from build123d import *

# Parameters (mm, degrees)
F1_DEPTH = 3.8
F2_DEPTH = 7.6
F3_R     = 7
F4_R     = 3
F5_R     = 4
F6_R     = 1.7


with BuildPart() as f1:
    # F0 (on Front) → F1 (new body)
    with BuildSketch(Plane.XZ):
        with BuildLine():
            Line((19.1431716898, 4.4253403938), (8.1440456616, 19.750261103))
            Line((8.1440456616, 19.750261103), (-6.1453692615, 19.750261103))
            add(Edge.make_bspline(
                [(-6.1453692615, 19.750261103), (-9.4334975883, 18.3276780648), (-20.4694799737, 9.4077816301), (-28.441204782, -7.9211202874), (-28.3713925064, -15.033986271), (-24.9090821352, -17.6588842502), (-22.1613161266, -18.3001520287)],
                knots=[0, 0, 0, 0, 0.3043807241, 0.630499808, 0.8116691041, 1, 1, 1, 1], degree=3))
            add(Edge.make_bspline(
                [(-22.1613161266, -18.3001520287), (-20.4320557503, -18.7037231321), (-13.2463438928, -20.672034694), (-7.2728786379, -21.7751605126)],
                knots=[0, 0, 0, 0, 14.676670933, 14.676670933, 14.676670933, 14.676670933], degree=3))
            add(Edge.make_bspline(
                [(-7.2728786379, -21.7751605126), (-10.7580149359, -20.0565494265), (-8.7832123206, -14.063103822), (-8.03378309, -11.3945532964), (-9.0233562514, -8.6834942922)],
                knots=[0, 0, 0, 0, 0.5245717937, 1, 1, 1, 1], degree=3))
            add(Edge.make_bspline(
                [(-9.0233562514, -8.6834942922), (-10.6191516402, -5.3268720907), (-10.1119981872, -0.4332128436), (-8.8609410373, 1.4029428946), (-3.6260034076, 1.6703835883), (-3.5176839858, 0), (-3.8980361515, -1.1065827018)],
                knots=[0, 0, 0, 0, 0.3686579414, 0.5465668413, 0.8102724675, 1, 1, 1, 1], degree=3))
            ThreePointArc((-3.8980361515, -1.1065827018), (0.6821136218, 1.3926973088), (5.0296685697, -1.4922530361))
            add(Edge.make_bspline(
                [(8.4968951944, -8.8667105614), (10.512974474, -6.6020334922), (10.6178822415, 0.1333355699), (9.2147437469, 1.7017312358), (5.6166367294, 1.6619292411), (4.4507364715, 0.9827180402), (4.4928646091, -0.16227164), (5.0296685697, -1.4922530361)],
                knots=[0, 0, 0, 0, 0.3364900582, 0.4892530829, 0.6935980051, 0.8097848409, 0.9832063696, 0.9832063696, 0.9832063696, 0.9832063696], degree=3))
            add(Edge.make_bspline(
                [(8.4968951944, -8.8667105614), (8.93450925, -9.375769436), (10.8149022533, -11.1384536985), (13.7340780615, -11.7891050671), (15.0382904123, -11.7891050671)],
                knots=[0.3188114686, 0.3188114686, 0.3188114686, 0.3188114686, 0.5009211334, 1, 1, 1, 1], degree=3))
            Line((15.0382904123, -11.7891050671), (19.1431716898, -11.7891050671))
            Line((19.1431716898, -11.7891050671), (19.1431716898, 4.4253403938))
        make_face()
        with BuildLine():
            ThreePointArc((-22.1613161266, -14.6834942922), (-25.1613161266, -11.6834942922), (-22.1613161266, -8.6834942922))
            Line((-22.1613161266, -8.6834942922), (-14.628011294, -8.6834942922))
            ThreePointArc((-14.628011294, -8.6834942922), (-11.628011294, -11.6834942922), (-14.628011294, -14.6834942922))
            Line((-14.628011294, -14.6834942922), (-22.1613161266, -14.6834942922))
        make_face(mode=Mode.SUBTRACT)
        with BuildLine():
            ThreePointArc((3.2729445693, 16.7312547565), (6.2729445693, 13.7312547565), (3.2729445693, 10.7312547565))
            Line((3.2729445693, 10.7312547565), (-4.2603602633, 10.7312547565))
            ThreePointArc((-4.2603602633, 10.7312547565), (-7.2603602633, 13.7312547565), (-4.2603602633, 16.7312547565))
            Line((-4.2603602633, 16.7312547565), (3.2729445693, 16.7312547565))
        make_face(mode=Mode.SUBTRACT)
    extrude(amount=F1_DEPTH)

    # F0 (on Front) → F2 (join)
    with BuildSketch(Plane.XZ):
        with BuildLine():
            add(Edge.make_bspline(
                [(-7.2728786379, -21.7751605126), (-10.7580149359, -20.0565494265), (-8.7832123206, -14.063103822), (-8.03378309, -11.3945532964), (-9.0233562514, -8.6834942922)],
                knots=[0, 0, 0, 0, 0.5245717937, 1, 1, 1, 1], degree=3))
            add(Edge.make_bspline(
                [(-7.2728786379, -21.7751605126), (-3.8634845801, -22.4047767321), (-0.848995576, -22.7525474742), (0.5306684761, -22.3666733306)],
                knots=[14.676670933, 14.676670933, 14.676670933, 14.676670933, 23.053476109, 23.053476109, 23.053476109, 23.053476109], degree=3))
            ThreePointArc((0.5306684761, -22.3666733306), (1.3315647917, -21.7109648486), (1.3916492908, -20.6776312264))
            Line((1.3916492908, -20.6776312264), (-4.2720503639, -5.4112309833))
            ThreePointArc((-4.2720503639, -5.4112309833), (-4.5685146727, -3.2168998843), (-3.8980361515, -1.1065827018))
            add(Edge.make_bspline(
                [(-9.0233562514, -8.6834942922), (-10.6191516402, -5.3268720907), (-10.1119981872, -0.4332128436), (-8.8609410373, 1.4029428946), (-3.6260034076, 1.6703835883), (-3.5176839858, 0), (-3.8980361515, -1.1065827018)],
                knots=[0, 0, 0, 0, 0.3686579414, 0.5465668413, 0.8102724675, 1, 1, 1, 1], degree=3))
        make_face()
        with BuildLine():
            add(Edge.make_bspline(
                [(6.7479446556, -6.068916612), (7.1641658841, -6.9684223917), (7.730783303, -7.9755233328), (8.4968951944, -8.8667105614)],
                knots=[0, 0, 0, 0, 0.3188114686, 0.3188114686, 0.3188114686, 0.3188114686], degree=3))
            add(Edge.make_bspline(
                [(8.4968951944, -8.8667105614), (10.512974474, -6.6020334922), (10.6178822415, 0.1333355699), (9.2147437469, 1.7017312358), (5.6166367294, 1.6619292411), (4.4507364715, 0.9827180402), (4.4928646091, -0.16227164), (5.0296685697, -1.4922530361)],
                knots=[0, 0, 0, 0, 0.3364900582, 0.4892530829, 0.6935980051, 0.8097848409, 0.9832063696, 0.9832063696, 0.9832063696, 0.9832063696], degree=3))
            ThreePointArc((5.0296685697, -1.4922530361), (5.1193553392, -1.6928196399), (5.2002361796, -1.8970963366))
            Line((5.2002361796, -1.8970963366), (6.7479446556, -6.068916612))
        make_face()
    extrude(amount=F2_DEPTH)

    # F3
    f3_edges = [f1.edges().sort_by_distance(p)[0] for p in [
        (-6.145369, -1.9, 19.750261),
    ]]
    fillet(f3_edges, radius=F3_R)

    # F4
    f4_edges = [f1.edges().sort_by_distance(p)[0] for p in [
        (8.144046, -1.9, 19.750261),
    ]]
    fillet(f4_edges, radius=F4_R)

    # F5
    f5_edges = [f1.edges().sort_by_distance(p)[0] for p in [
        (19.143172, -1.9, 4.42534),
    ]]
    fillet(f5_edges, radius=F5_R)

    # F6
    f6_edges = [f1.edges().sort_by_distance(p)[0] for p in [
        (19.143172, -1.9, -11.789105),
    ]]
    fillet(f6_edges, radius=F6_R)


solid = f1.part
Work out the finished part from the listing and answer in its coordinate system (mm). A direction names the side the tool comes from. Round coordinates to 2 decimals unless told otherwise and drop trailing zeros. Use one line per item in the form item = value. Start each with the question number.
(1) Flat-ended cylindrical pins translate along their axes: P1, Ø3, axis at y = -6, z = -1.5, coming from the -X side; P2, Ø12.5, axis at x = -11, z = 7.5, coming from the -Y side; P3, Ø1.1, axis at x = -2, y = -2, coming from the -Z side; P4, Ø6, axis at x = 2.5, z = -10.5, coming from the +Y side. Find the tip coordinate at first contact, or state that the pin passes through.
(2) Find section A-A on y = -0.75. Give the number of separate pieces and of enclosed holes in the cut face, and give its area (3 significant figures).
(3) Determine the mould class of faces 6 (the face through (-18, -2, -8.683)), 7 (the face through (-1, -2, 16.731)), 8 (the face through (-4.3, 0, -1.2)), 9 (the face through (1, -2, 19.75)) for opening direction Z: +Z half, -Z half, draft (parallel to the pull), parting line (faces both ways), or undercut.
(4) Consider line 1 (Y direction, x = -13, z = 0); line 2 (Z direction, x = -18, y = -0.75); line 3 (Z direction, x = -24.5, y = -0.25). Determine where each line is inside the solid, lowest interval first.
(5) Which of the six approach directions +Z, -Z, +X, -X, +Y, -Y give full straight-line access (tool end or side, diameter ignored) to faces 1 (the face through (6.272, -1.873, 13.797)), 2 (the face through (16, -2, -11.789)), 3 (the face through (1.325, -3.747, -21.724)), 4 (the face through (5.96, -3.75, -3.95)), 5 (the face through (-6, -7.6, -10))?
Answer list:
q1.P1 = -10.19
q1.P2 = -3.8
q1.P3 = -22.52
q1.P4 = through
q2.separate_pieces = 1
q2.enclosed_holes = 2
q2.area = 1,120 mm^2
q3.face_6 = undercut
q3.face_7 = undercut
q3.face_8 = draft
q3.face_9 = +Z half
q4.line_1 = -3.8 to 0
q4.line_2 = -19.35 to -14.68, -8.68 to 9.84
q4.line_3 = -17.48 to -13.56, -9.8 to -0.15
q5.face_1 = +Y, -Y
q5.face_2 = -Z, +X, +Y, -Y
q5.face_3 = +X, +Y, -Y
q5.face_4 = -Z, +Y, -Y
q5.face_5 = +Z, -Z, +X, -X, -Y
